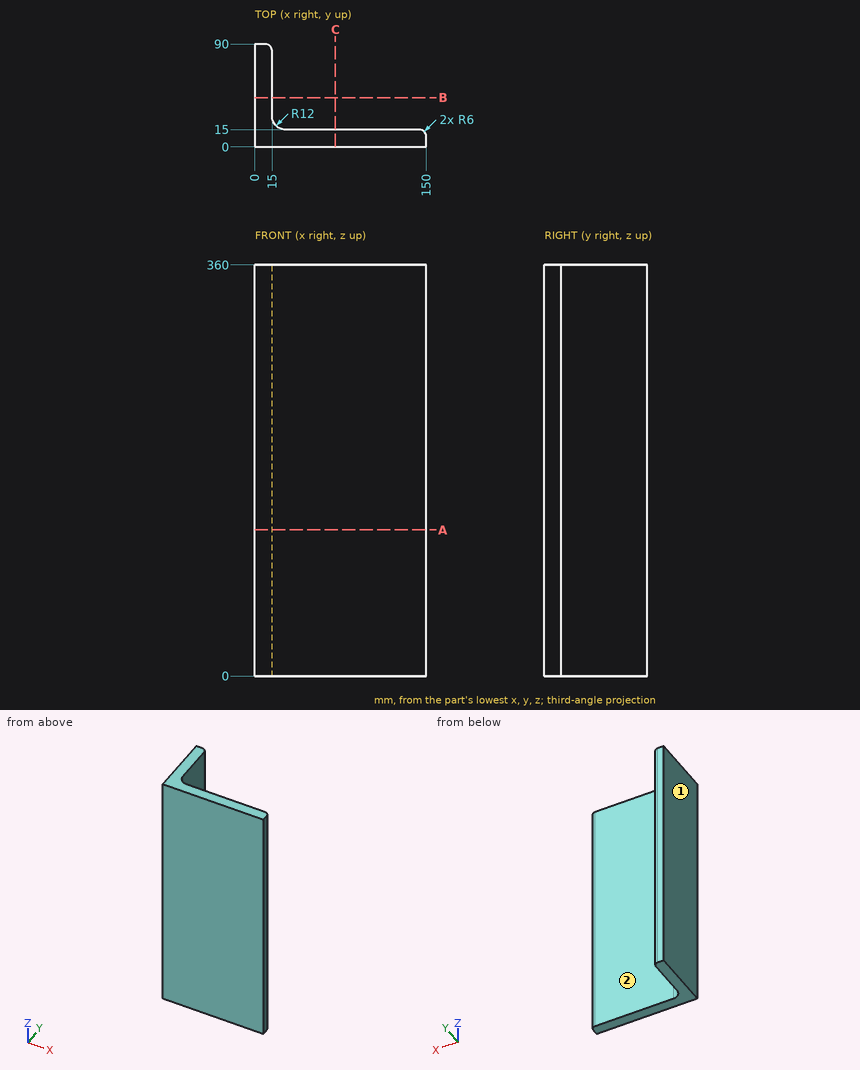
Could you check a few things on this drawing? It's one solid part, dimensions in mm from its lowest x, y, z. A direction names the side the tool comes from. Round coordinates to 2 decimals unless told otherwise and drop trailing zeros. Order: outer loops, then holes, each group sorted by start corner. A loop starts at its lowest first (then second) coordinate and runs counter-clockwise, first axis right, second up.
Q1. Which directions (+Z, -Z, +X, -X, +Y, -Y) give clear straight access to the entire face, cutting with the end or side of a thin tool? Please do the marked faces 1 and 2.
Geometry says:
face 1: +Z, -Z, -X, +Y, -Y
face 2: +Z, -Z, +X, +Y
Q2. Please list where these lines run through material, in increasing order: probe 1 along Y at (x, z) = (120, 306.5); probe 2 along X at (y, z) = (10, 75).
Geometry says:
probe 1: y = 0 to 15
probe 2: x = 0 to 149.92
Q3. Imagine slicing it at B-B, the plane y = 43. List the corners of the cut face in (x, z) for me, then the cut area to 3 significant figures.
Geometry says:
outline: (0, 0) - (15, 0) - (15, 360) - (0, 360) - close
area: 5,400 mm2
Q4. I'm going to push flat-ended pins straight in: P1, Ø3, axis at y = 56, z = 297.5, coming from the +X side; P2, Ø8, axis at x = 63, z = 155, coming from the +Y side. Where does each tip first touch, or does it pass through?
Geometry says:
P1: stops at x = 15
P2: stops at y = 15
Q5. Imagine slicing it at A-A, the plane z = 128. List the corners of the cut face in (x, y) for me.
Geometry says:
outline: (0, 0) - (150, 0) - (150, 9) arc R6 ccw to (144, 15) - (27, 15) arc R12 cw to (15, 27) - (15, 84) arc R6 ccw to (9, 90) - (0, 90) - close
